Study the drawing (mm; zero at the part's minimum x, y, z) and answer. A direction names the side the tool comes from. Give positions to 0.01 mm unless a question says otherwise; leave off trailing zeros. Write each loop counter-clockwise with the first axis right and the second up, starting at its lowest first coordinate (ties: lowest second). Pieces come first, ordered by that corner, then holes. Notation, with made-up numbers: M 57.5,-3.5 L 98.5,-3.5 A24 cw 98.5,32.5 Z; hole C 28.5,2 d10. An arc over 180 degrees is marked long. Use a Markdown table: item, result. Add a question column.
Item 1: A cutting plane is placed at D-D on x = 12.5. Determine the outline of the cut face in (y, z).
Item 2: A cutting plane is placed at A-A on x = 19.5. Determine the outline of the cut face in (y, z), then the cut area to 3 significant figures.
Item 3: The mould has two halves that part along Z. Classify the marked faces 3, 4, 5 and 6: pulls with the +Z half, pulls with the -Z half, needs draft (parallel to the pull), parting line crosses it, or undercut.
Item 4: A cutting plane is placed at B-B on y = 2.75. Determine the outline of the cut face in (x, z).
Item 5: For the marked faces 1 and 2, determine the directions among +Z, -Z, +X, -X, +Y, -Y from which every point of the face is accessible in a straight line to the end or side of a thin tool.
Item 6: Consider probe 1 along Z at (x, y) = (12, 0.8) (1 decimal); probe 2 along Z at (x, y) = (12.25, 1.2); probe 3 along Z at (x, y) = (2, 2.15) (1 decimal). Determine where each line is inside the solid, lowest interval first. Write a range as [from, to].
Item 7: Given P1, Ø3, axis at x = 12, z = 15.5, coming from the +Y side, flat-ended and moving along its own axis, determine where the tip first touches the part or whether it passes through.
Item 8: A cutting plane is placed at C-C on z = 15. Determine the outline of the cut face in (x, y).
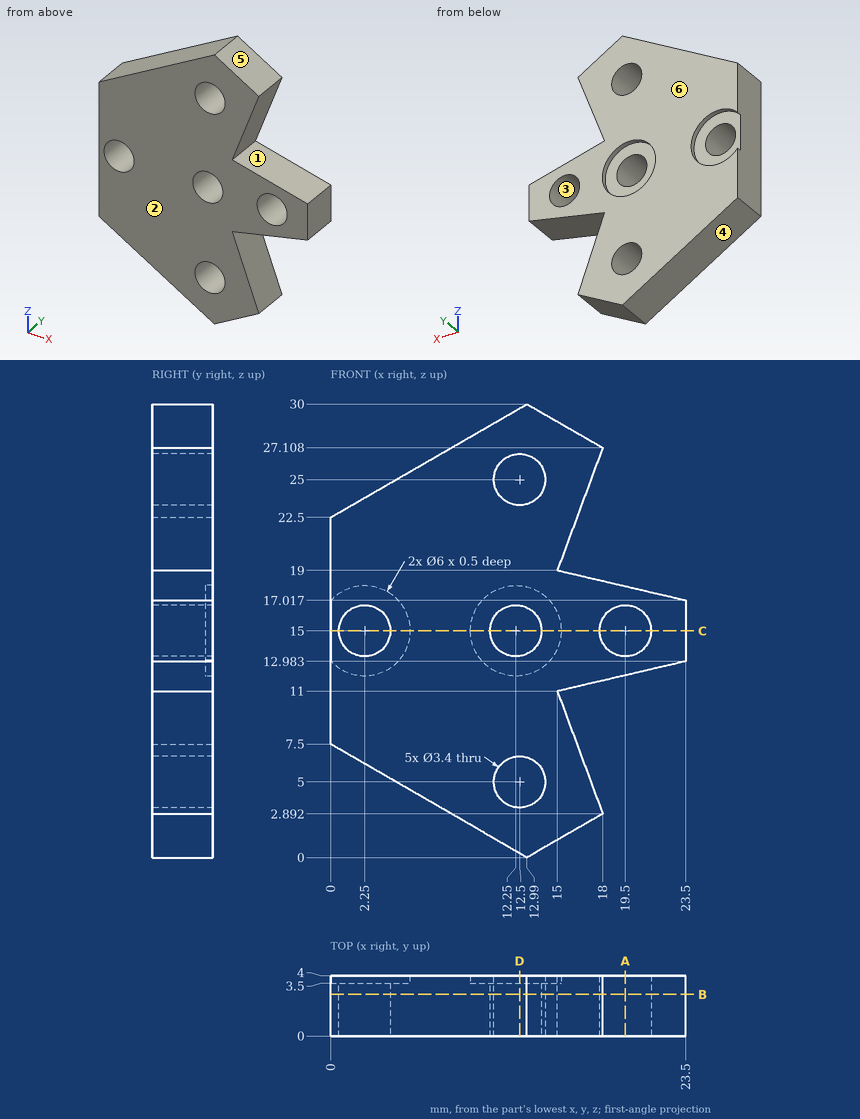
Filled in:
| question | item | result |
|---|---|---|
| 1 | outline | M 0,0.28 L 4,0.28 L 4,3.3 L 0,3.3 Z; M 0,6.7 L 4,6.7 L 4,12.01 L 3.5,12.01 L 3.5,13.32 L 0,13.32 Z; M 0,16.68 L 3.5,16.68 L 3.5,17.99 L 4,17.99 L 4,23.3 L 0,23.3 Z; M 0,26.7 L 4,26.7 L 4,29.72 L 0,29.72 Z |
| 2 | outline | M 0,12.05 L 4,12.05 L 4,13.3 L 0,13.3 Z; M 0,16.7 L 4,16.7 L 4,17.95 L 0,17.95 Z |
| 2 | area | 10.0 mm² |
| 3 | face 3 | undercut |
| 3 | face 4 | pulls with the -Z half |
| 3 | face 5 | pulls with the +Z half |
| 3 | face 6 | needs draft |
| 4 | outline | M 0,7.5 L 12.99,0 L 18,2.89 L 15,11 L 23.5,12.98 L 23.5,17.02 L 15,19 L 18,27.11 L 12.99,30 L 0,22.5 Z; hole C 2.25,15 d3.4; hole C 12.25,15 d3.4; hole C 12.5,5 d3.4; hole C 12.5,25 d3.4; hole C 19.5,15 d3.4 |
| 5 | face 1 | +X, +Y, -Y |
| 5 | face 2 | +Z, -Z, +X, -X, -Y |
| 6 | probe 1 | [0.6, 3.4], [6.6, 13.3], [16.7, 23.4], [26.6, 29.4] |
| 6 | probe 2 | [0.43, 3.32], [6.68, 13.3], [16.7, 23.32], [26.68, 29.57] |
| 6 | probe 3 | [6.3, 13.3], [16.7, 23.7] |
| 7 | P1 | y = 3.5 |
| 8 | outline | M 0,0 L 0.55,0 L 0.55,3.5 L 0,3.5 Z; M 3.95,0 L 10.55,0 L 10.55,3.5 L 9.25,3.5 L 9.25,4 L 5.25,4 L 5.25,3.5 L 3.95,3.5 Z; M 13.95,0 L 17.8,0 L 17.8,4 L 15.25,4 L 15.25,3.5 L 13.95,3.5 Z; M 21.2,0 L 23.5,0 L 23.5,4 L 21.2,4 Z |
